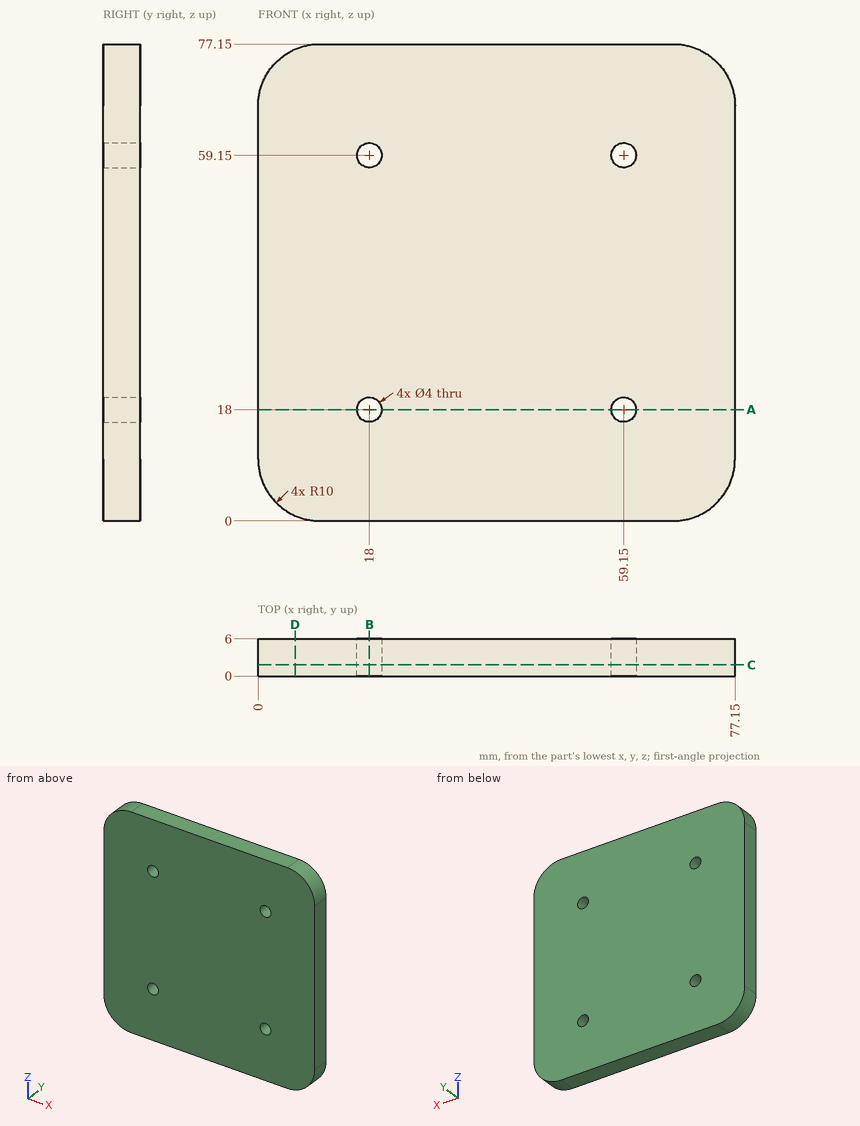
Geometry check sheet. Reference: drawing and pictorial views, mm from the part's lowest x, y, z. Round coordinates to 2 decimals unless told otherwise and drop trailing zeros. Write each loop counter-clockwise with the first axis right and the second up, starting at its lowest first coordinate (ties: lowest second). Pieces come first, ordered by that corner, then holes.
1. Section check D-D on x = 6. Enter the section's corners in (y, z), plus the area to 3 significant figures.
2. Section check B-B on x = 18. Enter the section's corners in (y, z).
3. Section check A-A on z = 18. Enter the section's corners in (x, y), plus the area to 3 significant figures.
4. Section check C-C on y = 1.8. Enter the section's corners in (x, z), plus the area to 3 significant figures.
5. Scan lines: L1, parallel to Z at x = 18, y = 2.35; L2, parallel to X at y = 3.35, z = 60. Record each from-to range of solid material in increasing order.
Answer:
1. outline: (0, 0.83) - (6, 0.83) - (6, 76.32) - (0, 76.32) - close
1. area: 453 mm2
2. outline: (0, 0) - (6, 0) - (6, 16) - (0, 16) - close; (0, 20) - (6, 20) - (6, 57.15) - (0, 57.15) - close; (0, 61.15) - (6, 61.15) - (6, 77.15) - (0, 77.15) - close
3. outline: (0, 0) - (16, 0) - (16, 6) - (0, 6) - close; (20, 0) - (57.15, 0) - (57.15, 6) - (20, 6) - close; (61.15, 0) - (77.15, 0) - (77.15, 6) - (61.15, 6) - close
3. area: 415 mm2
4. outline: (0, 10) arc R10 ccw to (10, 0) - (67.15, 0) arc R10 ccw to (77.15, 10) - (77.15, 67.15) arc R10 ccw to (67.15, 77.15) - (10, 77.15) arc R10 ccw to (0, 67.15) - close; hole circle Ø4 at (18, 18); hole circle Ø4 at (18, 59.15); hole circle Ø4 at (59.15, 18); hole circle Ø4 at (59.15, 59.15)
4. area: 5,820 mm2
5. L1: z = 0 to 16, 20 to 57.15, 61.15 to 77.15
5. L2: x = 0 to 16.19, 19.81 to 57.34, 60.96 to 77.15
